Can you work these out from the model? Positions are in its coordinate system, mm. A direction names the side the tool comes from. Round coordinates to 2 decimals unless told otherwise and drop trailing zeros. Loops run counter-clockwise (first coordinate to the right, second up) from the corner with the lowest first, then second, coordinate; pieces in that order, holes last.
from build123d import *

# Parameters (mm, degrees)
F0_W     = 80
F0_H     = 60
F0_R     = 3
F1_DEPTH = 25
F2_T     = -1.5


with BuildPart() as f1:
    # F0 (on Top) → F1 (new body)
    with BuildSketch(Plane.XY):
        with Locations((15.248706, 10.717015)):
            Rectangle(F0_W, F0_H)
        with Locations((49.856115, -13.597123)):
            Circle(F0_R, mode=Mode.SUBTRACT)
    extrude(amount=F1_DEPTH)

    # F2
    f2_openings = [f1.faces().sort_by_distance(p)[0] for p in [
        (15.043643, 10.861085, 25),
    ]]
    offset(amount=F2_T, openings=f2_openings)


solid = f1.part
(1) If we mould it in two halves opening along Y, with no side actions, what happens to faces 1 (the flat face through (15, -19.283, 12)), 2 (the flat face through (15, 40.717, 12)), 3 (the flat face through (6, -18, 25)), 4 (the cylindrical face through (52.8, -17, 13.1))? For each: released by +Y, released by -Y, zero draft, split by the parting line, or undercut.
Worked answers:
face 1: released by -Y
face 2: released by +Y
face 3: zero draft
face 4: undercut
(2) Will this pin go through, and if not, where does the flat tip stop? P1, Ø17, axis at x = 19, y = -3, coming from the +Z side.
Worked answers:
P1: stops at z = 1.5
(3) If we section it at A-A, the plane x = -9: List the corners of the cut face in (y, z) for me.
Worked answers:
outline: (-19.28, 0) - (40.72, 0) - (40.72, 25) - (39.22, 25) - (39.22, 1.5) - (-17.78, 1.5) - (-17.78, 25) - (-19.28, 25) - close
(4) For faces 5 (the cylindrical face through (49.206, -16.526, 12.325)), 6 (the flat face through (-23.251, 10, 13)), which set-ups out of +Z, -Z, +X, -X, +Y, -Y let a thin tool reach every point of the face, with its end or its side?
Worked answers:
face 5: +Z, -Z
face 6: +Z
(5) If we section it at B-B, the plane z = 13.75: List the corners of the cut face in (x, y) for me.
Worked answers:
outline: (-24.75, -19.28) - (55.25, -19.28) - (55.25, 40.72) - (-24.75, 40.72) - close; hole (-23.25, -17.78) - (48.2, -17.78) arc R4.5 cw (long way) to (53.75, -11.34) - (53.75, 39.22) - (-23.25, 39.22) - close; hole circle Ø6 at (49.86, -13.6); hole (51.51, -17.78) - (53.75, -17.78) - (53.75, -15.85) arc R4.5 cw to start
(6) If I drill on line 1 (Y direction, x = 14, z = 10.5); line 2 (X direction, y = 33.5, z = 20.25); line 3 (X direction, y = -15, z = 20.25), over which ranges is the centre line in solid material (lowest first)?
Worked answers:
line 1: y = -19.28 to -17.78, 39.22 to 40.72
line 2: x = -24.75 to -23.25, 53.75 to 55.25
line 3: x = -24.75 to -23.25, 45.58 to 47.2, 52.51 to 55.25
(7) If we section it at C-C, the plane y = 13.5: List the corners of the cut face in (x, z) for me, then the cut area to 4 significant figures.
Worked answers:
outline: (-24.75, 0) - (55.25, 0) - (55.25, 25) - (53.75, 25) - (53.75, 1.5) - (-23.25, 1.5) - (-23.25, 25) - (-24.75, 25) - close
area: 190.5 mm2
